from build123d import *

# Parameters (mm, degrees)
F1_DEPTH = 39.37
F3_D     = 8.89
F5_D     = 1.905
F7_DEPTH = 16.002


with BuildPart() as f1:
    # F0 (on Right) → F1 (new body)
    with BuildSketch(Plane.YZ):
        with BuildLine():
            Line((-1.27, 0), (0, 0))
            ThreePointArc((0, 0), (-4.572, 6.35), (0, 12.7))
            Line((0, 12.7), (-1.27, 12.7))
            ThreePointArc((-1.27, 12.7), (-5.334, 6.35), (-1.27, 0))
        make_face()
    extrude(amount=F1_DEPTH)

    # F3 (through all)
    with Locations(Plane(origin=(0, 0, 0), x_dir=(1, 0, 0), z_dir=(0, 1, 0))):
        with Locations((19.05, -6.35)):
            Hole(F3_D / 2)

    # F5 (through all)
    with Locations(Plane(origin=(0, 0, 0), x_dir=(1, 0, 0), z_dir=(0, 1, 0))):
        with Locations((6.35, -6.35)):
            Hole(F5_D / 2)

    # F6 (on Front) → F7 (cut)
    with BuildSketch(Plane.XZ):
        with BuildLine():
            Line((29.464, 8.89), (29.464, 6.35))
            Line((29.464, 6.35), (29.464, 3.81))
            ThreePointArc((29.464, 3.81), (30.2895, 2.9845), (31.115, 3.81))
            Line((31.115, 3.81), (31.115, 6.35))
            Line((31.115, 6.35), (31.115, 8.89))
            ThreePointArc((31.115, 8.89), (30.2895, 9.7155), (29.464, 8.89))
        make_face()
    extrude(amount=F7_DEPTH, mode=Mode.SUBTRACT)


solid = f1.part
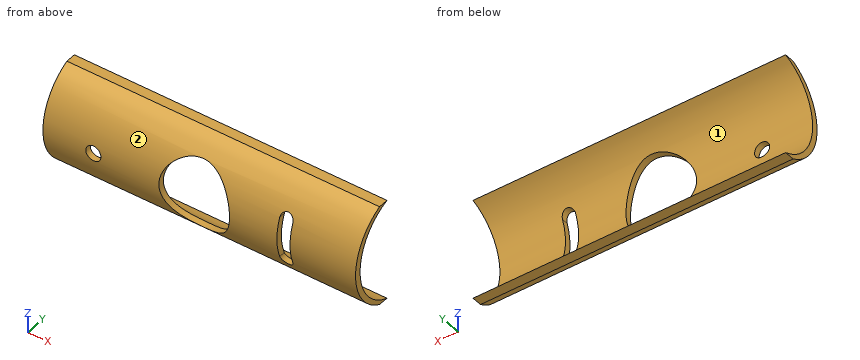
Design review of the part built by this model. Coordinates are the model's own, in mm. Face numbers are marked on the shaded views. Give positions to 0.01 mm unless a question says otherwise; leave off trailing zeros. Loops run counter-clockwise (first coordinate to the right, second up) from the corner with the lowest first, then second, coordinate; pieces in that order, holes last. Notation, with made-up numbers: (10, 36) -> (46, 36) arc R9 ccw to (46, 46) -> close; hole circle Ø2 at (-33.5, -13). An arc over 180 degrees is marked (long way). One line per question, with ' | ' between items. Start each with the question number.
(1) We need section A-A (z = 6.35). State the section outline as (x, y) points (1 decimal), and give its area (3 significant figures).
(2) We need section B-B (y = -1.65). State the section outline as (x, z) points.
(3) Insertion check: P1, Ø1.5, axis at x = 15, y = -4.5, coming from the +Z side; P2, Ø3, axis at x = 12.5, y = -4, coming from the -Z side. Each pin has a flat end and moves straight along its axis. Give the tip position at first contact, or say it passes through.
(4) For line 1 (X direction, y = -4.6, z = 5.5) (3 decimals); line 2 (Z direction, x = 8, y = -1.2); line 3 (Z direction, x = 18, y = -1.95), list the stretches that pass through material, from the lowest coordinate up.
(5) Draft analysis for pull direction Z (two halves, no side actions). For the marked faces 1 and 2, state which applies: +Z half, -Z half, draft (parallel to the pull), parting line (faces both ways), or undercut.
(6) We need section D-D (x = 10.5). State the section outline as (y, z) points.
The answers:
1) outline: (0, -5.3) -> (5.4, -5.3) -> (5.4, -4.6) -> (0, -4.6) -> close; (7.3, -5.3) -> (14.6, -5.3) -> (14.6, -4.6) -> (7.3, -4.6) -> close; (23.5, -5.3) -> (29.5, -5.3) -> (29.5, -4.6) -> (23.5, -4.6) -> close; (31.1, -5.3) -> (39.4, -5.3) -> (39.4, -4.6) -> (31.1, -4.6) -> close | area: 20.5 mm^2
2) outline: (0, 0.19) -> (39.37, 0.19) -> (39.37, 0.82) -> (0, 0.82) -> close; (0, 11.88) -> (39.37, 11.88) -> (39.37, 12.51) -> (0, 12.51) -> close
3) P1: stops at z = 10.78 | P2: stops at z = 0.73
4) line 1: x = 0 to 5.92, 6.78 to 14.687, 23.413 to 29.464, 31.115 to 39.37 | line 2: z = 0 to 0.54, 12.16 to 12.7 | line 3: z = 0.36 to 1.04, 11.66 to 12.34
5) face 1: undercut | face 2: parting line
6) outline: (-1.27, 0) -> (0, 0) arc R6.7 cw to (0, 12.7) -> (-1.27, 12.7) arc R6.99 ccw to start
